Design review of the part built by this model. Coordinates are the model's own, in mm. A direction names the side the tool comes from. Coordinates: 2 decimals unless noted, no trailing zeros. Order: outer loops, then holes, each group sorted by start corner. A loop starts at its lowest first (then second) coordinate and runs counter-clockwise, first axis right, second up. Notation, with made-up numbers: M 65,5 L 109,5 A26 cw 109,40 Z; hole C 48,65.5 d3. An arc over 180 degrees is marked long. Answer in a Markdown table with one row per item.
from build123d import *
from build123d.topology import SkipClean

# Parameters (mm, degrees)
SKETCH_1_R               = 18
EXTRUDE_1_DEPTH          = 1.5
EXTRUDE_2_DEPTH          = 6
EXTRUDE_2_DEPTH_BACK     = 6.5
SKETCH_2_R               = 20
SKETCH_2_R_2             = 18
CUT_EXTRUDE_START        = 1.5
SKETCH_6_R               = 1
CUT_EXTRUDE_4_DEPTH      = 8
CUT_EXTRUDE_5_DEPTH      = 30.393876913
CUT_EXTRUDE_5_DEPTH_BACK = 30.393876913
CUT_EXTRUDE_6_DEPTH      = 1.5
EXTRUDE_START            = 8
EXTRUDE_3_DEPTH          = 6.5


with BuildPart() as part:
    # 草图1 → 凸台-拉伸1 (new body)
    with BuildSketch(Plane(origin=(0, 0, 0), x_dir=(1, 0, 0), z_dir=(0, 1, 0))):
        with Locations(Location((0, 0, 0), (0, 0, 270))):
            Circle(SKETCH_1_R)
    extrude(amount=EXTRUDE_1_DEPTH)

    # 草图2 → 凸台-拉伸2 (add, two sides: drawn at the far end of the back side and taken through both)
    with BuildSketch(Plane(origin=(0, 0, 0), x_dir=(1, 0, 0), z_dir=(0, 1, 0)).offset(-EXTRUDE_2_DEPTH_BACK)):
        with Locations(Location((0, 0, 0), (0, 0, 270))):
            Circle(SKETCH_2_R)
        with Locations(Location((0, 0, 0), (0, 0, 270))):
            Circle(SKETCH_2_R_2, mode=Mode.SUBTRACT)
    extrude(amount=EXTRUDE_2_DEPTH + EXTRUDE_2_DEPTH_BACK)

    # 扫描2: sweep along a curve in space
    with SkipClean():  # the faces are left unmerged after this step: merging them gives an invalid solid
        with BuildLine() as sweep_2_path:
            ThreePointArc((0, 6, 18), (12.727922061, 6, 12.727922061), (18, 6, 0))
            ThreePointArc((18, 6, 0), (12.727922061, 6, -12.727922061), (0, 6, -18))
            ThreePointArc((0, 6, -18), (-12.727922061, 6, -12.727922061), (-18, 6, 0))
            ThreePointArc((-18, 6, 0), (-12.727922061, 6, 12.727922061), (0, 6, 18))
        # 草图5 → 扫描2 (sweep)
        with BuildSketch(Plane.XY):
            Polygon((-20, 6), (-18, 6), (-18, 8), align=None)
        sweep(path=sweep_2_path.line)

    # 草图6 → 切除-拉伸4 (cut)
    with SkipClean():  # the faces are left unmerged after this step: merging them gives an invalid solid
        with BuildSketch(Plane(origin=(0, 0, 0), x_dir=(1, 0, 0), z_dir=(0, 1, 0)).offset(CUT_EXTRUDE_START)):
            with Locations(Location((0, -12.5, 0), (0, 0, 270))):
                Circle(SKETCH_6_R)
            with Locations(Location((0, 12.5, 0), (0, 0, 270))):
                Circle(SKETCH_6_R)
        extrude(amount=-CUT_EXTRUDE_4_DEPTH, mode=Mode.SUBTRACT)

    # 草图7 → 切除-拉伸5 (cut, two sides: drawn at the far end of the back side and taken through both)
    with BuildSketch(Plane(origin=(0, 0, 0), x_dir=(1, 0, 0), z_dir=(0, 1, 0)).offset(-CUT_EXTRUDE_5_DEPTH_BACK)):
        with BuildLine():
            Line((-19.843134833, -2.5), (-15.07554347, -2.5))
            Line((-15.07554347, -2.5), (-15.07554347, 2.5))
            Line((-15.07554347, 2.5), (-19.843134833, 2.5))
            ThreePointArc((-19.843134833, 2.5), (-20, 0), (-19.843134833, -2.5))
        make_face()
        with BuildLine():
            Line((15.07554347, 2.5), (15.07554347, -2.5))
            Line((15.07554347, -2.5), (19.843134833, -2.5))
            ThreePointArc((19.843134833, -2.5), (20, 0), (19.843134833, 2.5))
            Line((19.843134833, 2.5), (15.07554347, 2.5))
        make_face()
    extrude(amount=CUT_EXTRUDE_5_DEPTH + CUT_EXTRUDE_5_DEPTH_BACK, mode=Mode.SUBTRACT)

    # 草图8 → 切除-拉伸6 (cut)
    with SkipClean():  # the faces are left unmerged after this step: merging them gives an invalid solid
        with BuildSketch(Plane(origin=(0, 0, 0), x_dir=(1, 0, 0), z_dir=(0, 1, 0)).offset(CUT_EXTRUDE_START)):
            with BuildLine():
                Line((10.606601706, 12.020815293), (12.001158233, 13.41537182))
                ThreePointArc((12.001158233, 13.41537182), (12.727922049, 12.727922074), (13.415371797, 12.001158259))
                Line((13.415371797, 12.001158259), (12.020815268, 10.606601731))
                ThreePointArc((12.020815268, 10.606601731), (10.606601706, 10.606601706), (10.606601706, 12.020815293))
            make_face()
            with BuildLine():
                Line((12.020815268, -10.606601731), (13.415371797, -12.001158259))
                ThreePointArc((13.415371797, -12.001158259), (12.727922049, -12.727922074), (12.001158233, -13.41537182))
                Line((12.001158233, -13.41537182), (10.606601706, -12.020815293))
                ThreePointArc((10.606601706, -12.020815293), (10.606601706, -10.606601706), (12.020815268, -10.606601731))
            make_face()
            with BuildLine():
                Line((-10.606601706, -12.020815293), (-12.001158233, -13.41537182))
                ThreePointArc((-12.001158233, -13.41537182), (-12.727922049, -12.727922074), (-13.415371797, -12.001158259))
                Line((-13.415371797, -12.001158259), (-12.020815268, -10.606601731))
                ThreePointArc((-12.020815268, -10.606601731), (-10.606601706, -10.606601706), (-10.606601706, -12.020815293))
            make_face()
            with BuildLine():
                Line((-12.020815268, 10.606601731), (-13.415371797, 12.001158259))
                ThreePointArc((-13.415371797, 12.001158259), (-12.727922049, 12.727922074), (-12.001158233, 13.41537182))
                Line((-12.001158233, 13.41537182), (-10.606601706, 12.020815293))
                ThreePointArc((-10.606601706, 12.020815293), (-10.606601706, 10.606601706), (-12.020815268, 10.606601731))
            make_face()
        extrude(amount=-CUT_EXTRUDE_6_DEPTH, mode=Mode.SUBTRACT)

    # 草图9 → 凸台-拉伸3 (add)
    with SkipClean():  # the faces are left unmerged after this step: merging them gives an invalid solid
        with BuildSketch(Plane(origin=(0, 0, 0), x_dir=(1, 0, 0), z_dir=(0, 1, 0)).offset(EXTRUDE_START)):
            with BuildLine():
                Line((12.020815268, -10.606601731), (13.415371797, -12.001158259))
                ThreePointArc((13.415371797, -12.001158259), (13.906042657, -11.428997228), (14.372329608, -10.836795727))
                Line((14.372329608, -10.836795727), (13.081475446, -9.545941553))
                ThreePointArc((13.081475446, -9.545941553), (9.545941558, -9.545941548), (9.545941537, -13.081475443))
                Line((9.545941537, -13.081475443), (10.8367957, -14.372329629))
                ThreePointArc((10.8367957, -14.372329629), (11.428997201, -13.906042679), (12.001158233, -13.41537182))
                Line((12.001158233, -13.41537182), (10.606601718, -12.020815281))
                ThreePointArc((10.606601718, -12.020815281), (10.606601731, -10.606601731), (12.020815268, -10.606601731))
            make_face()
            with BuildLine():
                Line((-10.606601718, -12.020815281), (-12.001158233, -13.41537182))
                ThreePointArc((-12.001158233, -13.41537182), (-11.428997201, -13.906042679), (-10.8367957, -14.372329629))
                Line((-10.8367957, -14.372329629), (-9.545941547, -13.081475453))
                ThreePointArc((-9.545941547, -13.081475453), (-9.545941551, -9.545941542), (-13.081475462, -9.545941556))
                Line((-13.081475462, -9.545941556), (-14.372329609, -10.836795726))
                ThreePointArc((-14.372329609, -10.836795726), (-13.906042657, -11.428997227), (-13.415371797, -12.001158259))
                Line((-13.415371797, -12.001158259), (-12.020815281, -10.606601718))
                ThreePointArc((-12.020815281, -10.606601718), (-10.606601718, -10.606601718), (-10.606601718, -12.020815281))
            make_face()
            with BuildLine():
                Line((10.606601718, 12.020815281), (12.001158233, 13.41537182))
                ThreePointArc((12.001158233, 13.41537182), (11.428997201, 13.906042679), (10.8367957, 14.372329629))
                Line((10.8367957, 14.372329629), (9.545941547, 13.081475453))
                ThreePointArc((9.545941547, 13.081475453), (9.545941551, 9.545941542), (13.081475462, 9.545941556))
                Line((13.081475462, 9.545941556), (14.372329609, 10.836795726))
                ThreePointArc((14.372329609, 10.836795726), (13.906042657, 11.428997227), (13.415371797, 12.001158259))
                Line((13.415371797, 12.001158259), (12.020815281, 10.606601718))
                ThreePointArc((12.020815281, 10.606601718), (10.606601718, 10.606601718), (10.606601718, 12.020815281))
            make_face()
            with BuildLine():
                Line((-12.020815268, 10.606601731), (-13.415371797, 12.001158259))
                ThreePointArc((-13.415371797, 12.001158259), (-13.906042657, 11.428997228), (-14.372329608, 10.836795727))
                Line((-14.372329608, 10.836795727), (-13.081475446, 9.545941553))
                ThreePointArc((-13.081475446, 9.545941553), (-9.545941558, 9.545941548), (-9.545941537, 13.081475443))
                Line((-9.545941537, 13.081475443), (-10.8367957, 14.372329629))
                ThreePointArc((-10.8367957, 14.372329629), (-11.428997201, 13.906042679), (-12.001158233, 13.41537182))
                Line((-12.001158233, 13.41537182), (-10.606601718, 12.020815281))
                ThreePointArc((-10.606601718, 12.020815281), (-10.606601731, 10.606601731), (-12.020815268, 10.606601731))
            make_face()
        extrude(amount=-EXTRUDE_3_DEPTH)


solid = part.part
(1) Insertion check: pin 1 Ø1.5 at (x, y) = (9, -3) entering from -Z; pin 2 Ø2.5 at (x, y) = (16.5, 1) entering from +Z; pin 3 Ø1 at (x, z) = (4, 0.5) entering from -Y; pin 4 Ø12 at (x, z) = (13, 11.5) entering from -Y. Each pin has a flat end and moves straight along its axis. Give the tip position at first contact, or say it passes through.
Return value:
| item | result |
|---|---|
| pin 1 | stops at z = -18.22 |
| pin 2 | stops at z = 12.94 |
| pin 3 | stops at y = 0 |
| pin 4 | stops at y = -6.5 |
(2) For faces 4 (the flat face through (18, 1, 2.5)), 5 (the flat face through (-13.736, 4.796, -10.2)), 6 (the flat face through (-12.708, 4.056, -11.294)), list the 3-axis set-ups (+Z, -Z, +X, -X, +Y, -Y) from which the entire face can be reached by the end or side of a thin tool; tool diameter is ignored.
Return value:
| item | result |
|---|---|
| face 4 | +X, +Y, -Y |
| face 5 | +Y |
| face 6 | +Y, -Y |
(3) Draft analysis for pull direction X (two halves, no side actions). For faces 1 (the flat face through (-15.076, 1, 0)), 2 (the cylindrical face through (0, 0, 20)), 3 (the cylindrical face through (-9.507, 4.796, 9.585)), state which applies: pulls with the +X half, pulls with the -X half, needs draft (parallel to the pull), parting line crosses it, or undercut.
Return value:
| item | result |
|---|---|
| face 1 | pulls with the -X half |
| face 2 | parting line crosses it |
| face 3 | undercut |
(4) For line 1 along Z through (x, y) = (0.5, -3.5); line 2 along X through (y, z) = (0.9, 12.5); line 3 along Z through (x, y) = (13, 4.5), list the stretches that pass through material, from the lowest coordinate up. Write a range as from..to.
Return value:
| item | result |
|---|---|
| line 1 | z = -19.99..-17.99, 17.99..19.99 |
| line 2 | x = -15.61..-12.95, -11.09..-1, 1..11.09, 12.95..15.61 |
| line 3 | z = -15.2..-12.45, -11.59..-9.47, 9.47..11.59, 12.45..15.2 |
(5) Add section B-B, the plane y = 4.25. Give the number of separate pieces and of enclosed holes in the cut face, and give its area (3 significant figures).
Return value:
| item | result |
|---|---|
| separate pieces | 2 |
| enclosed holes | 4 |
| area | 275 mm2 |
(6) Add section C-C, the plane z = -2. Give the boundary of the cut face in (x, y), and give its area (3 significant figures).
Return value:
| item | result |
|---|---|
| outline | M -15.08,0 L 15.08,0 L 15.08,1.5 L -15.08,1.5 Z |
| area | 45.2 mm2 |
